Build history of the part. All positions in model axes, mm. A direction names the side the tool comes from. Give positions to 0.01 mm unless a question says otherwise; leave off trailing zeros. Order: outer loops, then holes, each group sorted by start corner. A loop starts at its lowest first (then second) coordinate and runs counter-clockwise, first axis right, second up. Notation, with made-up numbers: (-5, 16) - (23, 16) arc R18 cw to (23, 26) - close; hole circle Ø6 at (-38.75, -5.75). An arc over 180 degrees is marked (long way). Use a Markdown table: item, result.
Autodesk Inventor part; units mm, degrees
ref_plane "YZ Plane" through (0, 0, 0) normal (1, 0, 0) x (0, 1, 0)
ref_plane "XZ Plane" through (0, 0, 0) normal (0, 1, 0) x (-1, 0, 0)
ref_plane "XY Plane" through (0, 0, 0) normal (0, 0, 1) x (1, 0, 0)
sketch "Sketch1" plane through (0, 0, 0) normal (0, 0, 1) x (1, 0, 0)
  circle A0 centre (0, 0) radius 6.35
  dimension "d0" = 12.7
extrude "Extrusion1" add sketch "Sketch1" along normal blind 1.905
sketch "Sketch2" plane through (0, 0, 1.905) normal (0, 0, 1) x (1, 0, 0)
  circle A0 centre (0, 0) radius 6.35
  circle A1 centre (0, 0) radius 3.4925
  dimension "d3" = 6.985
extrude "Extrusion2" add sketch "Sketch2" along normal blind 1.905 contours A1
sketch "Sketch3" plane through (0, 0, 3.81) normal (0, 0, 1) x (1, 0, 0)
  circle A0 centre (0, 0) radius 3.4925
  circle A1 centre (0, 0) radius 6.35
  circle A2 centre (0, 0) radius 6.35
extrude "Extrusion3" add sketch "Sketch3" along normal blind 1.27 contours A0 | A1
sketch "Sketch4" plane through (0, 0, 5.08) normal (0, 0, 1) x (1, 0, 0)
  circle A0 centre (0, 0) radius 6.35
  circle A1 centre (0, 0) radius 3.175
  dimension "d8" = 6.35
extrude "Extrusion4" cut sketch "Sketch4" against normal through all contours A1
properties part number "Pnewmatic Screw Part 2 1764"
1) Two-plate mould, pull along Z, no slides. Class faces 3 (the cylindrical face through (-0.69, -3.1, 2.58)), 4 (the flat face through (-2, 3, 5.08)), 5 (the cylindrical face through (-0.455, -3.463, 2.844)): +Z half, -Z half, draft (parallel to the pull), parting line (faces both ways), or undercut.
Computed:
| item | result |
|---|---|
| face 3 | draft |
| face 4 | +Z half |
| face 5 | undercut |
2) Pin check, flat tips, straight feed: P1, Ø1, axis at y = 3.5, z = 1, coming from the -X side; P2, Ø2, axis at x = -1.5, z = 0.5, coming from the +Y side. Stop position of each tip, or through.
Computed:
| item | result |
|---|---|
| P1 | stops at x = -5.6 |
| P2 | stops at y = 6.33 |
3) Tool access for faces 1 (the flat face through (3, -3, 1.905)), 2 (the cylindrical face through (-1.38, 6.2, 0.94)): list every direction of +Z, -Z, +X, -X, +Y, -Y with a clear straight run to the whole face (end or side of a thin tool).
Computed:
| item | result |
|---|---|
| face 1 | none |
| face 2 | +Z, -Z |
4) Slice it at D-D (y = -4.75). Write the cut outline in (x, z) (3 decimals), and give its area (3 significant figures).
Computed:
| item | result |
|---|---|
| outline | (-4.214, 0) - (4.214, 0) - (4.214, 1.905) - (-4.214, 1.905) - close; (-4.214, 3.81) - (4.214, 3.81) - (4.214, 5.08) - (-4.214, 5.08) - close |
| area | 26.8 mm² |
5) Wall check: line 1 (Y direction, x = 0, z = 1.65) (3 decimals); line 2 (Y direction, x = 0, z = 2.6) (1 decimal); line 3 (Z direction, x = 1.75, y = 5.75) (3 decimals). Give the ranges that are in metal, low to high. Write a range as from..to.
Computed:
| item | result |
|---|---|
| line 1 | y = -6.35..-3.175, 3.175..6.35 |
| line 2 | y = -3.5..-3.2, 3.2..3.5 |
| line 3 | z = 0..1.905, 3.81..5.08 |
